CAD build for the part. Positions are in the model's coordinates, mm. Face numbers are marked on the shaded views. Round coordinates to 2 decimals unless told otherwise and drop trailing zeros. Loops run counter-clockwise (first coordinate to the right, second up) from the corner with the lowest first, then second, coordinate; pieces in that order, holes last. Notation, with made-up numbers: (72.5, 38.5) - (85.5, 38.5) arc R22 cw to (85.5, 49.5) - close; hole circle Ø2 at (79.5, -2.75). An arc over 180 degrees is marked (long way). One line per question, with ' | ' between items.
```python
from build123d import *

# Parameters (mm, degrees)
EXTRUDE17_DEPTH = 1.6129
SKETCH19_R      = 3.6195
EXTRUDE19_DEPTH = 4.2291
SKETCH20_R      = 0.46355
SKETCH20_R_2    = 1.27
EXTRUDE20_DEPTH = 5.2291
SKETCH21_R      = 2.44475
EXTRUDE21_DEPTH = 1.1557
SKETCH22_R      = 2.286
EXTRUDE22_DEPTH = 2.3368


with BuildPart() as part:
    # Sketch18 → Extrude17 (new body)
    with BuildSketch(Plane(origin=(0, 0, 0), x_dir=(1, 0, 0), z_dir=(0, 1, 0))):
        with BuildLine():
            Line((-14.34305969, 1.923991942), (-2.13741415, 2.921))
            ThreePointArc((-2.13741415, 2.921), (0, 3.6195), (2.13741415, 2.921))
            Line((2.13741415, 2.921), (14.34305969, 1.923991942))
            ThreePointArc((14.34305969, 1.923991942), (16.1163, 0), (14.34305969, -1.923991942))
            Line((14.34305969, -1.923991942), (2.13741415, -2.921))
            ThreePointArc((2.13741415, -2.921), (0, -3.6195), (-2.13741415, -2.921))
            Line((-2.13741415, -2.921), (-14.34305969, -1.923991942))
            ThreePointArc((-14.34305969, -1.923991942), (-16.1163, 0), (-14.34305969, 1.923991942))
        make_face()
    extrude(amount=EXTRUDE17_DEPTH)

    # Sketch19 → Extrude19 (add)
    with BuildSketch(Plane(origin=(0, 1.6129, 0), x_dir=(1, 0, 0), z_dir=(0, 1, 0))):
        Circle(SKETCH19_R)
    extrude(amount=-EXTRUDE19_DEPTH)

    # Sketch20 → Extrude20 (cut, through all)
    with BuildSketch(Plane(origin=(0, 1.6129, 0), x_dir=(1, 0, 0), z_dir=(0, 1, 0))):
        with Locations((-14.1859, 0)):
            Circle(SKETCH20_R)
        Circle(SKETCH20_R_2)
        with Locations((-4.6609, 0)):
            Circle(SKETCH20_R)
        with Locations((-6.5659, 0)):
            Circle(SKETCH20_R)
        with Locations((-8.4709, 0)):
            Circle(SKETCH20_R)
        with Locations((-10.3759, 0)):
            Circle(SKETCH20_R)
        with Locations((-12.2809, 0)):
            Circle(SKETCH20_R)
    extrude20 = extrude(amount=-EXTRUDE20_DEPTH, mode=Mode.SUBTRACT)

    # Mirror1: Extrude20 across plane
    add(extrude20.mirror(Plane(origin=(0, 0, 0), x_dir=(0, 0, 1), z_dir=(1, 0, 0))), mode=Mode.SUBTRACT)

    # Sketch21 → Extrude21 (cut)
    with BuildSketch(Plane(origin=(0, 1.6129, 0), x_dir=(1, 0, 0), z_dir=(0, 1, 0))):
        Circle(SKETCH21_R)
    extrude(amount=-EXTRUDE21_DEPTH, mode=Mode.SUBTRACT)

    # Sketch22 → Extrude22 (cut)
    with BuildSketch(Plane.XZ.offset(2.6162)):
        Circle(SKETCH22_R)
    extrude(amount=-EXTRUDE22_DEPTH, mode=Mode.SUBTRACT)


solid = part.part
```
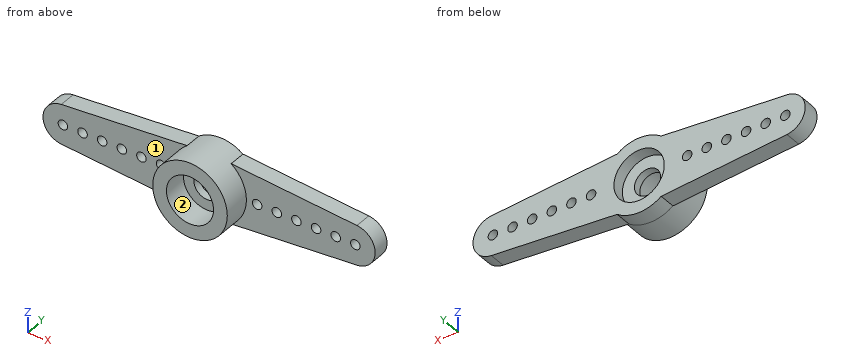
(1) Probe L1, parallel to Y at x = 13.5, z = -1.25; L2, parallel to Z at x = 0, y = 0.85; L3, parallel to Z at x = 2, y = -0.95. List the from-to ranges inside material, lowest first.
Results found:
L1: y = 0 to 1.61 | L2: z = -3.62 to -2.44, 2.44 to 3.62 | L3: z = -3.02 to -1.11, 1.11 to 3.02
(2) Cut at B-B, the plane x = 0. Write the cut outline in (y, z).
Results found:
outline: (-2.62, -3.62) - (1.61, -3.62) - (1.61, -2.44) - (0.46, -2.44) - (0.46, -1.27) - (-0.28, -1.27) - (-0.28, -2.29) - (-2.62, -2.29) - close; (-2.62, 2.29) - (-0.28, 2.29) - (-0.28, 1.27) - (0.46, 1.27) - (0.46, 2.44) - (1.61, 2.44) - (1.61, 3.62) - (-2.62, 3.62) - close
(3) Drop flat-ended pins along their axis: P1, Ø3, axis at x = -10, z = 0.5, coming from the -Y side; P2, Ø4, axis at x = 0, z = 0, coming from the +Y side; P3, Ø3.5, axis at x = 0, z = -0.5, coming from the -Y side. Give the stop position or say it passes through.
Results found:
P1: stops at y = 0 | P2: stops at y = 0.46 | P3: stops at y = -0.28
(4) Cut at C-C, the plane y = -0.85. Write the cut outline in (x, z).
Results found:
outline: circle Ø7.24 at (0, 0); hole circle Ø4.57 at (0, 0)
(5) Two-plate mould, pull along Z, no slides. Class the marked faces 1 and 2: released by +Z, released by -Z, zero draft, split by the parting line, or undercut.
Results found:
face 1: zero draft | face 2: undercut
(6) Cut at D-D, the plane x = -6.5. Write the cut outline in (y, z), then the cut area to 3 significant figures.
Results found:
outline: (0, -2.56) - (1.61, -2.56) - (1.61, -0.46) - (0, -0.46) - close; (0, 0.46) - (1.61, 0.46) - (1.61, 2.56) - (0, 2.56) - close | area: 6.79 mm²
(7) Cut at A-A, the plane z = -0.75. Write the cut outline in (x, y), then the cut area to 3 significant figures.
Results found:
outline: (-15.96, 0) - (-3.54, 0) - (-3.54, -2.62) - (-2.16, -2.62) - (-2.16, -0.28) - (-1.02, -0.28) - (-1.02, 0.46) - (-2.33, 0.46) - (-2.33, 1.61) - (-15.96, 1.61) - close; (1.02, -0.28) - (2.16, -0.28) - (2.16, -2.62) - (3.54, -2.62) - (3.54, 0) - (15.96, 0) - (15.96, 1.61) - (2.33, 1.61) - (2.33, 0.46) - (1.02, 0.46) - close | area: 53.0 mm²
